For this review, take the finished solid that the model builds, in its own axes (mm). A direction names the side the tool comes from. Give positions to 0.01 mm unless a question says otherwise; leave off trailing zeros. Loops run counter-clockwise (first coordinate to the right, second up) from the corner with the lowest first, then second, coordinate; pieces in that order, holes last.
```python
from build123d import *

# Parameters (mm, degrees)
EXTRUSION1_DEPTH = 148


with BuildPart() as part:
    # Esquisse1 → Extrusion1 (new body, symmetric)
    with BuildSketch(Plane.XY):
        Polygon((-0.75, 0), (-0.75, 10), (0.75, 10), (0.75, 0), (5, 0), (12.207425429, -3.47174577), (10.905520765, -6.174530306), (10.004592586, -5.740562084), (10.872529029, -3.938705727), (4.771707198, -1), (-4.771707198, -1), (-10.872529029, -3.938705727), (-10.004592586, -5.740562084), (-10.905520765, -6.174530306), (-12.207425429, -3.47174577), (-5, 0), align=None)
    extrude(amount=EXTRUSION1_DEPTH, both=True)


solid = part.part
```
Q1. For pin 1 Ø1 at (x, y) = (4, 1) entering from +Z; pin 2 Ø8 at (y, z) = (2.5, -62) entering from +X; pin 3 Ø5 at (y, z) = (3, -32) entering from -X; pin 4 Ø2 at (x, z) = (-2.5, -43) entering from +Y, all flat-tipped, find the tip position at first contact; note any pin that passes through.
Answers:
pin 1: passes through
pin 2: stops at x = 8.11
pin 3: stops at x = -0.75
pin 4: stops at y = 0
Q2. Mouldability with a two-part tool opening along X and no side actions: class faces 4 (the flat face through (8.55, -1.71, 2.07)), 5 (the flat face through (0, -1, 2)), 6 (the flat face through (0, 0, 148)) as +X half, -X half, draft (parallel to the pull), parting line (faces both ways), or undercut.
Answers:
face 4: +X half
face 5: undercut
face 6: draft
Q3. Consider section B-B on y = 6.25. Give the boundary of the cut face in (x, z), plus the area to 3 significant figures.
Answers:
outline: (-0.75, -148) - (0.75, -148) - (0.75, 148) - (-0.75, 148) - close
area: 444 mm2
Q4. Machinability: for faces 1 (the flat face through (-0.75, 5, 2)), 2 (the flat face through (0.75, 5, 2)), 3 (the flat face through (0, 0, -148)), which of the approach directions +Z, -Z, +X, -X, +Y, -Y give a long, thin tool a straight path to every point of the face, cutting with its end or side? Answer none if there is none.
Answers:
face 1: +Z, -Z, -X, +Y
face 2: +Z, -Z, +X, +Y
face 3: -Z, +X, -X, +Y, -Y
Q5. For probe 1 along X at (y, z) = (1, -38); probe 2 along X at (y, z) = (-2.75, -134); probe 3 along Y at (x, z) = (-4.75, -87.5), list the stretches that pass through material, from the lowest coordinate up.
Answers:
probe 1: x = -0.75 to 0.75
probe 2: x = -10.71 to -8.4, 8.4 to 10.71
probe 3: y = -1 to 0
Q6. Consider section A-A on z = 33.5. Give the boundary of the cut face in (x, y).
Answers:
outline: (-12.21, -3.47) - (-10.91, -6.17) - (-10, -5.74) - (-10.87, -3.94) - (-4.77, -1) - (4.77, -1) - (10.87, -3.94) - (10, -5.74) - (10.91, -6.17) - (12.21, -3.47) - (5, 0) - (0.75, 0) - (0.75, 10) - (-0.75, 10) - (-0.75, 0) - (-5, 0) - close
